Could you check a few things on this drawing? It's one solid part, dimensions in mm from its lowest x, y, z. A direction names the side the tool comes from. Give positions to 0.01 mm unless a question says otherwise; leave off trailing zeros. Loops run counter-clockwise (first coordinate to the right, second up) from the corner with the lowest first, then second, coordinate; pieces in that order, holes last. Notation, with made-up numbers: (85, 39.25) - (128, 39.25) arc R16 ccw to (128, 54.25) - close; hole circle Ø8 at (-29, 29.25). An arc over 180 degrees is marked (long way). Use a Markdown table: item, result.
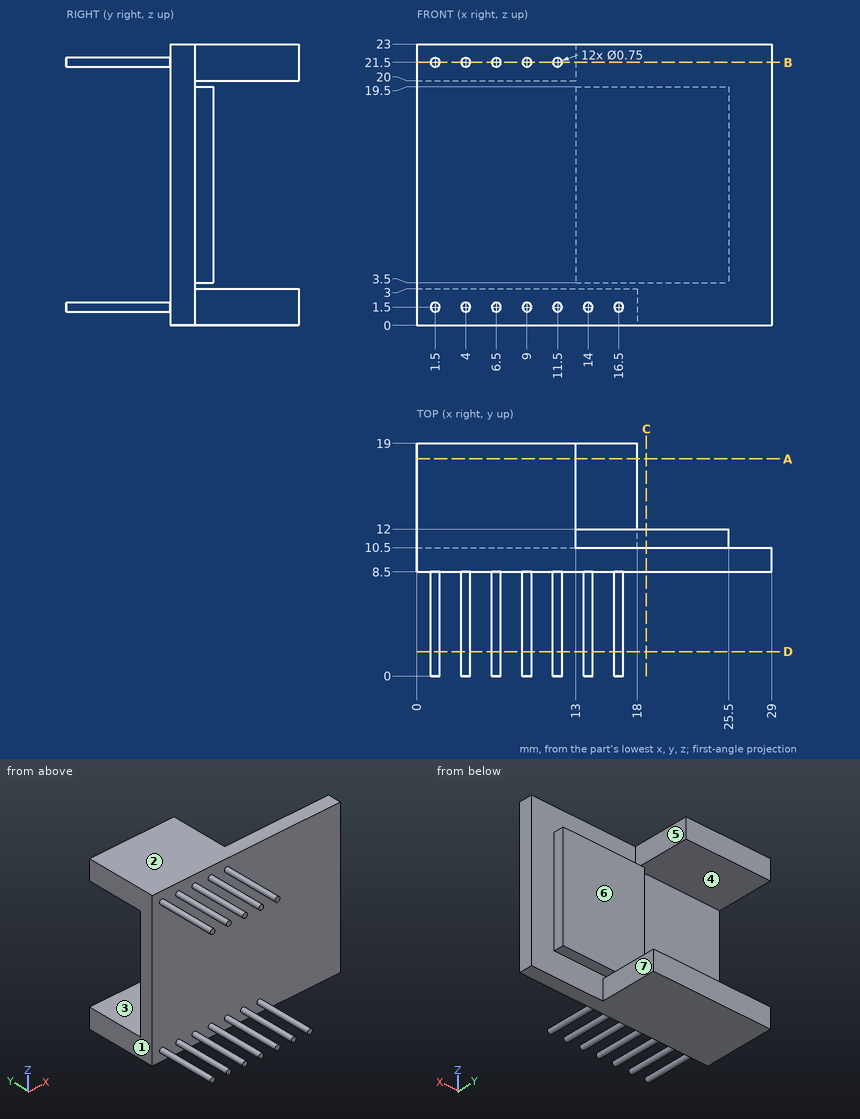
(1) We'd pull the mould along Z, two halves only. Please class the marked faces 1, 2 and 3: pulls with the +Z half, pulls with the -Z half, needs draft (parallel to the pull), parting line crosses it, or undercut.
A:
| item | result |
|---|---|
| face 1 | needs draft |
| face 2 | pulls with the +Z half |
| face 3 | undercut |
(2) Suppose I cut it at B-B on z = 21.5. Write out the boundary of the cut face in (x, y) (3 decimals).
A:
| item | result |
|---|---|
| outline | (0, 8.5) - (1.125, 8.5) - (1.125, 0) - (1.875, 0) - (1.875, 8.5) - (3.625, 8.5) - (3.625, 0) - (4.375, 0) - (4.375, 8.5) - (6.125, 8.5) - (6.125, 0) - (6.875, 0) - (6.875, 8.5) - (8.625, 8.5) - (8.625, 0) - (9.375, 0) - (9.375, 8.5) - (11.125, 8.5) - (11.125, 0) - (11.875, 0) - (11.875, 8.5) - (29, 8.5) - (29, 10.5) - (13, 10.5) - (13, 19) - (0, 19) - close |
(3) Suppose I cut it at D-D on y = 2. Count the separate pieces of the cut face and the enclosed holes in it, plus the area to 3 significant figures.
A:
| item | result |
|---|---|
| separate pieces | 12 |
| enclosed holes | 0 |
| area | 5.30 mm2 |
(4) Will these pins go through, and if not, where does the flat tip stop? pin 1 (2.5 mm diameter, centred on x = 9, y = 15.5, fed in from -Z); pin 2 (3 mm diameter, centred on x = 7, y = 3.5, fed in from +Z) (3 decimals); pin 3 (7 mm diameter, centred on x = 9, z = 8.5, fed in from -Y); pin 4 (6 mm diameter, centred on y = 5, z = 4.5, fed in from +X) (3 decimals).
A:
| item | result |
|---|---|
| pin 1 | z = 0 |
| pin 2 | z = 21.875 |
| pin 3 | y = 8.5 |
| pin 4 | x = 16.875 |
(5) Suppose I cut it at A-A on y = 17.75. Write out the boundary of the cut face in (x, z).
A:
| item | result |
|---|---|
| outline | (0, 0) - (18, 0) - (18, 3) - (0, 3) - close; (0, 20) - (13, 20) - (13, 23) - (0, 23) - close |
(6) If I drill on line 1 (X direction, y = 3, z = 21.5) (3 decimals); line 2 (Z direction, x = 9, y = 11.5); line 3 (Y direction, x = 10, z = 7.5), over which ranges is the centre line in solid material (lowest first)?
A:
| item | result |
|---|---|
| line 1 | 1.125 to 1.875, 3.625 to 4.375, 6.125 to 6.875, 8.625 to 9.375, 11.125 to 11.875 |
| line 2 | 0 to 3, 20 to 23 |
| line 3 | 8.5 to 10.5 |
(7) Suppose I cut it at C-C on x = 18.75. Write out the boundary of the cut face in (y, z).
A:
| item | result |
|---|---|
| outline | (8.5, 0) - (10.5, 0) - (10.5, 3.5) - (12, 3.5) - (12, 19.5) - (10.5, 19.5) - (10.5, 23) - (8.5, 23) - close |
(8) On a 3-axis mill with a long thin cutter (end or side, diameter ignored), from which of +Z, -Z, +X, -X, +Y, -Y can I reach the whole of each face in a straight line? I mean the marked faces 4, 5, 6 and 7. Say none if no direction works.
A:
| item | result |
|---|---|
| face 4 | +X, -X, +Y |
| face 5 | +Z, +X, +Y |
| face 6 | +Z, +X, -X, +Y |
| face 7 | -Z, +X, +Y |
